```python
from build123d import *

# Parameters (mm, degrees)
SKETCH_2_W          = 40
SKETCH_2_H          = 25
EXTRUDE_1_DEPTH     = 4
SKETCH_3_R          = 1.5
CUT_EXTRUDE_1_DEPTH = 4


with BuildPart() as part:
    # 草图2 → 凸台-拉伸1 (new body)
    with BuildSketch(Plane.XY):
        Rectangle(SKETCH_2_W, SKETCH_2_H)
    extrude(amount=EXTRUDE_1_DEPTH)

    # 草图3 → 切除-拉伸1 (cut)
    with BuildSketch(Plane.XY.offset(4)):
        with Locations((-15, 8)):
            Circle(SKETCH_3_R)
        with Locations((0, 8)):
            Circle(SKETCH_3_R)
        with Locations(Location((15, 8, 0), (0, 0, 180))):
            Circle(SKETCH_3_R)
        with Locations((15, -8)):
            Circle(SKETCH_3_R)
        with Locations(Location((0, -8, 0), (0, 0, 180))):
            Circle(SKETCH_3_R)
        with Locations(Location((-15, -8, 0), (0, 0, 180))):
            Circle(SKETCH_3_R)
    extrude(amount=-CUT_EXTRUDE_1_DEPTH, mode=Mode.SUBTRACT)


solid = part.part
```
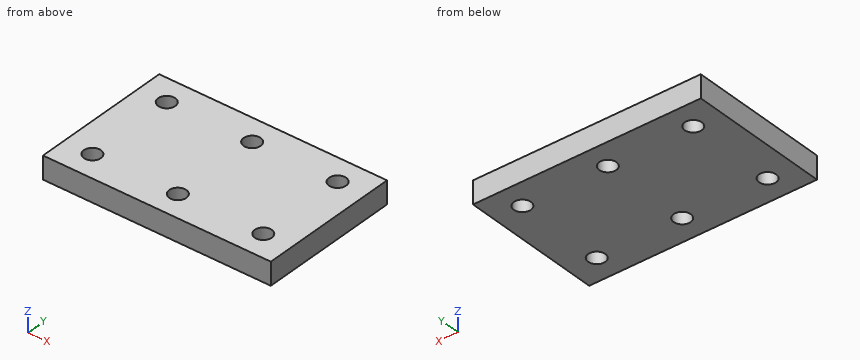
The listing builds one solid part. Answer for the finished solid, in the listing's coordinates (mm). Round coordinates to 2 decimals unless told otherwise and drop trailing zeros. Loops run counter-clockwise (first coordinate to the right, second up) from the corner with the lowest first, then second, coordinate; pieces in that order, holes last. Notation, with made-up numbers: (-29.5, 64) -> (-14.5, 64) arc R15 ccw to (-14.5, 89) -> close; hole circle Ø7 at (12, -6). An arc over 180 degrees is marked (long way). Use one line per item in the form item = value.
1. Find the intervals of material crossed by probe 1 along Y at (x, z) = (0, 1.85); probe 2 along X at (y, z) = (-7.75, 2.25); probe 3 along Y at (x, z) = (-16, 2.8), in increasing order. Write a range as [from, to].
Answer key:
probe_1 = [-12.5, -9.5], [-6.5, 6.5], [9.5, 12.5]
probe_2 = [-20, -16.48], [-13.52, -1.48], [1.48, 13.52], [16.48, 20]
probe_3 = [-12.5, -9.12], [-6.88, 6.88], [9.12, 12.5]
2. The part is cut by section C-C on y = 8. Determine the outline of the cut face in (x, z), and give its area (3 significant figures).
Answer key:
outline = (-20, 0) -> (-16.5, 0) -> (-16.5, 4) -> (-20, 4) -> close; (-13.5, 0) -> (-1.5, 0) -> (-1.5, 4) -> (-13.5, 4) -> close; (1.5, 0) -> (13.5, 0) -> (13.5, 4) -> (1.5, 4) -> close; (16.5, 0) -> (20, 0) -> (20, 4) -> (16.5, 4) -> close
area = 124 mm²
3. Flat-ended cylindrical pins translate along their axes: pin 1 Ø6 at (x, y) = (13.5, 6) entering from -Z; pin 2 Ø2.5 at (x, y) = (-15, -8) entering from +Z. Find the tip coordinate at first contact, or state that the pin passes through.
Answer key:
pin_1 = 0
pin_2 = through
4. The part is cut by section A-A on z = 1.1. Determine the outline of the cut face in (x, y), and give its area (3 significant figures).
Answer key:
outline = (-20, -12.5) -> (20, -12.5) -> (20, 12.5) -> (-20, 12.5) -> close; hole circle Ø3 at (-15, -8); hole circle Ø3 at (-15, 8); hole circle Ø3 at (0, -8); hole circle Ø3 at (0, 8); hole circle Ø3 at (15, -8); hole circle Ø3 at (15, 8)
area = 958 mm²
5. The part is cut by section B-B on x = 0. Determine the outline of the cut face in (y, z), and give its area (3 significant figures).
Answer key:
outline = (-12.5, 0) -> (-9.5, 0) -> (-9.5, 4) -> (-12.5, 4) -> close; (-6.5, 0) -> (6.5, 0) -> (6.5, 4) -> (-6.5, 4) -> close; (9.5, 0) -> (12.5, 0) -> (12.5, 4) -> (9.5, 4) -> close
area = 76.0 mm²
